The model under review builds one solid part; all positions refer to its coordinate system, in mm. Give positions to 0.01 mm unless a question says otherwise; leave off trailing zeros. Order: outer loops, then holes, each group sorted by start corner. A loop starts at its lowest first (then second) coordinate and runs counter-clockwise, first axis right, second up.
```python
from build123d import *

# Parameters (mm, degrees)
F1_DEPTH = 8
F2_SIZE  = 1
F3_D     = 6.6
F4_D     = 9
F5_D     = 3.3
F5_DEPTH = 4.35
F5_TIP   = 0.9914200214


with BuildPart() as f1:
    # F0 (on Top) → F1 (new body)
    with BuildSketch(Plane.XY):
        with BuildLine():
            Line((-127.7485371086, -120), (122.231243908, -120))
            ThreePointArc((122.231243908, -120), (129.8459043656, -116.8459043656), (133, -109.231243908))
            Line((133, -109.231243908), (133, 109.231243908))
            ThreePointArc((133, 109.231243908), (129.8459043656, 116.8459043656), (122.231243908, 120))
            Line((122.231243908, 120), (-127.7485371086, 120))
            ThreePointArc((-127.7485371086, 120), (-131.4618821303, 118.4618821303), (-133, 114.7485371086))
            Line((-133, 114.7485371086), (-133, -114.7485371086))
            ThreePointArc((-133, -114.7485371086), (-131.4618821303, -118.4618821303), (-127.7485371086, -120))
        make_face()
    extrude(amount=F1_DEPTH)

    # F2
    f2_edges = [f1.edges().sort_by_distance(p)[0] for p in [
        (-2.758647, -120, 8),
        (129.845904, -116.845904, 8),
        (133, 0, 8),
        (129.845904, 116.845904, 8),
        (-2.758647, 120, 8),
        (-131.461882, 118.461882, 8),
        (-133, 0, 8),
        (-131.461882, -118.461882, 8),
    ]]
    chamfer(f2_edges, length=F2_SIZE)

    # F3 (through all)
    with Locations(Plane(origin=(0, 0, 0), x_dir=(1, 0, 0), z_dir=(0, 0, -1))):
        with Locations((-51, 60), (-51, 20), (-51, -20), (-51, -60), (51, -60), (51, -20), (51, 20), (51, 60)):
            Hole(F3_D / 2)

    # F4 (through all)
    with Locations(Plane(origin=(0, 0, 0), x_dir=(1, 0, 0), z_dir=(0, 0, -1))):
        with Locations((-93, 80), (-93, -40), (93, -40), (93, 80)):
            Hole(F4_D / 2)

    # F5
    with Locations(Plane(origin=(0, 0, 0), x_dir=(1, 0, 0), z_dir=(0, 0, -1))):
        with Locations((-92.5, 88), (-92.5, 106.5), (92.5, 88), (92.5, 106.5), (92.5, -88), (92.5, -106.5), (-92.5, -88), (-92.5, -106.5)):
            Hole(F5_D / 2, depth=F5_DEPTH)
            with Locations((0, 0, -(F5_DEPTH + F5_TIP / 2))):  # 118° drill point
                Cone(0, F5_D / 2, F5_TIP, mode=Mode.SUBTRACT)


solid = f1.part
```
1. To check wall thickness, follow line 1 (X direction, y = -60, z = 4); line 2 (Y direction, x = 51, z = 6.75); line 3 (X direction, y = 40, z = 4.5). State the ranges of each line that lie inside material, in increasing order.
2. Take a section at A-A (y = 40). Write out the cut boundary in (x, z).
3. Take a section at B-B (y = -20). Write out the cut boundary in (x, z), and give its area (3 significant figures).
4. Insertion check: pin 1 (5.5 mm diameter, centred on x = 93, y = -80, fed in from +Z). The pin has a flat end and moves straight along its axis. Give the tip position at first contact, or say it passes through.
5. Draft analysis for pull direction Y (two halves, no side actions). For faces 1 (the cylindrical face through (96.32, -83.04, 4.06)), 2 (the flat face through (133, -2, 3)), 3 (the cylindrical face through (54.3, 19.9, 4.1)), 4 (the flat face through (-5, -120, 3)), state which applies: pulls with the +Y half, pulls with the -Y half, needs draft (parallel to the pull), parting line crosses it, or undercut.
Answer:
1. line 1: x = -133 to -54.3, -47.7 to 47.7, 54.3 to 133
1. line 2: y = -120 to -63.3, -56.7 to -23.3, -16.7 to 16.7, 23.3 to 56.7, 63.3 to 120
1. line 3: x = -133 to -97.5, -88.5 to 88.5, 97.5 to 133
2. outline: (-133, 0) - (-97.5, 0) - (-97.5, 8) - (-132, 8) - (-133, 7) - close; (-88.5, 0) - (88.5, 0) - (88.5, 8) - (-88.5, 8) - close; (97.5, 0) - (133, 0) - (133, 7) - (132, 8) - (97.5, 8) - close
3. outline: (-133, 0) - (-54.3, 0) - (-54.3, 8) - (-132, 8) - (-133, 7) - close; (-47.7, 0) - (47.7, 0) - (47.7, 8) - (-47.7, 8) - close; (54.3, 0) - (133, 0) - (133, 7) - (132, 8) - (54.3, 8) - close
3. area: 2,020 mm2
4. pin 1: passes through
5. face 1: undercut
5. face 2: needs draft
5. face 3: undercut
5. face 4: pulls with the -Y half
